Autodesk Inventor part; units mm, degrees
ref_plane "YZ Plane" through (0, 0, 0) normal (1, 0, 0) x (0, 1, 0)
ref_plane "XZ Plane" through (0, 0, 0) normal (0, 1, 0) x (-1, 0, 0)
ref_plane "XY Plane" through (0, 0, 0) normal (0, 0, 1) x (1, 0, 0)
sketch "Sketch1" plane through (0, 0, 0) normal (0, 0, 1) x (1, 0, 0)
  circle A0 centre (0, 0) radius 4.435
  circle A1 centre (0, 0) radius 7.46
  dimension "d0" = 8.87
  dimension "d1" = 14.92
extrude "Extrusion1" add sketch "Sketch1" along normal blind 11.34
sketch "Sketch2" plane through (0, 0, 0) normal (0, 1, 0) x (-1, 0, 0)
  line L0 (7.46, 11.34) -> (-7.46, 11.34)
  line L1 (-7.46, 0) -> (7.46, 0)
  line L2 (7.46, 11.34) -> (-7.46, 11.34)
  line L3 (0, 11.34) -> (-5.375, 11.34) construction
  line L4 (-7.46, 0) -> (-7.46, 8.5) construction
  line L5 (-7.46, 0) -> (-7.46, 11.34)
  arc A0 (-7.46, 8.5) -> (-5.375, 11.34) centre (-9.3123, 12.0453) ccw
  line L6 (-5.375, 11.34) -> (-7.46, 11.34)
  line L7 (-7.46, 11.34) -> (-7.46, 8.5)
  line L8 (0, 11.34) -> (0, 0)
  dimension "d4" = 5.375
  dimension "d5" = 8.5
  dimension "d6" = 4
revolve "Revolution1" cut sketch "Sketch2" angle 360 about axis through (0, 0, 11.34) along (0, 0, -1) contours A0 L5 L0
thread "Thread1"
sketch "Sketch3" plane through (0, 0, 0) normal (0, 0, -1) x (-1, 0, 0)
  circle A0 centre (0, 0) radius 4.435
  circle A1 centre (0, 0) radius 7.46
  line L0 (3.731, -6.46) -> (-3.731, -6.46)
  line L1 (3.731, 6.46) -> (-3.731, 6.46)
  line L2 (6.98, -2.6327) -> (6.98, 2.6327)
  line L3 (-6.98, -2.6327) -> (-6.98, 2.6327)
  dimension "d10" = 12.92
  dimension "d11" = 6.46
  dimension "d12" = 13.96
  dimension "d13" = 6.98
extrude "Extrusion2" cut sketch "Sketch3" against normal blind 2.6 contours A1 L2 | L1 A1 | A1 L0 | L3 A1
properties part number "BallBearingCone"
Design review of the part built by this model. Coordinates are the model's own, in mm. A direction names the side the tool comes from. Coordinates: 2 decimals unless noted, no trailing zeros. Loops run counter-clockwise (first coordinate to the right, second up) from the corner with the lowest first, then second, coordinate; pieces in that order, holes last. Notation, with made-up numbers: (-24.5, 40.25) -> (28.5, 40.25) arc R8 ccw to (28.5, 55.25) -> close; hole circle Ø6 at (-33.5, 67.25). An arc over 180 degrees is marked (long way). Answer as a JSON object with one key per item and string values.
Q1. Clearance check with flat-ended pins moving along their axes: pin 1 Ø4 at (x, z) = (-2.5, 8) entering from +Y; pin 2 Ø0.8 at (x, z) = (-1, 1.5) entering from +Y; pin 3 Ø4 at (x, z) = (4.5, 4.5) entering from -Y. State where each tip first meets the part, or that it passes through.
Answer block:
{"pin 1": "stops at y = 7.44", "pin 2": "stops at y = 6.46", "pin 3": "stops at y = -7.03"}
Q2. Take a section at B-B on y = 0. Give the boundary of the cut face in (x, z) (3 decimals), plus the area to 3 significant figures.
Answer block:
{"outline": "(-7.46, 2.6) -> (-6.98, 2.6) -> (-6.98, 0) -> (-4.435, 0) -> (-4.435, 11.34) -> (-5.375, 11.34) arc R4 cw to (-7.46, 8.5) -> close; (4.435, 0) -> (6.98, 0) -> (6.98, 2.6) -> (7.46, 2.6) -> (7.46, 8.5) arc R4 cw to (5.375, 11.34) -> (4.435, 11.34) -> close", "area": "58.2 mm^2"}
Q3. Tool access review of faces 5 (the flat face through (-6.98, 0, 1)), 6 (the flat face through (0, -6.46, 1)), 7 (the flat face through (0, 7, 2.6)): name each direction out of +Z, -Z, +X, -X, +Y, -Y from which nothing blocks a thin tool from reaching the whole face with its end or side.
Answer block:
{"face 5": "-Z, -X, +Y, -Y", "face 6": "-Z, +X, -X, -Y", "face 7": "-Z, +X, -X, +Y"}
Q4. Take a section at C-C on z = 8. Give the boundary of the cut face in (x, y) (3 decimals), plus the area to 3 significant figures.
Answer block:
{"outline": "circle Ø14.92 at (0, 0); hole circle Ø8.87 at (0, 0)", "area": "113 mm^2"}
Q5. To check wall thickness, follow L1, parallel to Y at x = 0, z = 6 (3 decimals); L2, parallel to Y at x = -3.5, z = 1.5; L3, parallel to X at y = -1, z = 3.5. State the ranges of each line that lie inside material, in increasing order.
Answer block:
{"L1": "y = -7.46 to -4.435, 4.435 to 7.46", "L2": "y = -6.46 to -2.72, 2.72 to 6.46", "L3": "x = -7.39 to -4.32, 4.32 to 7.39"}
Q6. Take a section at A-A on x = 0. Give the boundary of the cut face in (y, z) (3 decimals), plus the area to 3 significant figures.
Answer block:
{"outline": "(-7.46, 2.6) -> (-6.46, 2.6) -> (-6.46, 0) -> (-4.435, 0) -> (-4.435, 11.34) -> (-5.375, 11.34) arc R4 cw to (-7.46, 8.5) -> close; (4.435, 0) -> (6.46, 0) -> (6.46, 2.6) -> (7.46, 2.6) -> (7.46, 8.5) arc R4 cw to (5.375, 11.34) -> (4.435, 11.34) -> close", "area": "55.5 mm^2"}
Q7. The part is to be moulded in two halves that separate along X. For faces 1 (the flat face through (0, 6.46, 1)), 2 (the cylindrical face through (-0.971, -7.397, 5.135)), 3 (the flat face through (6.98, 0, 1)), 4 (the cylindrical face through (2.046, 3.935, 5.591)), say which applies: +X half, -X half, draft (parallel to the pull), parting line (faces both ways), or undercut.
Answer block:
{"face 1": "draft", "face 2": "parting line", "face 3": "+X half", "face 4": "undercut"}
